```python
from build123d import *

# Parameters (mm, degrees)
F1_DEPTH = 1.5


with BuildPart() as f1:
    # F0 (on Front) → F1 (new body)
    with BuildSketch(Plane.XZ):
        with BuildLine():
            ThreePointArc((6.841464, -4), (7.649321, -2.072079), (7.925, 0))
            ThreePointArc((7.925, 0), (7.649321, 2.072079), (6.841464, 4))
            ThreePointArc((6.841464, 4), (5.603821, 5.603821), (4, 6.841464))
            ThreePointArc((4, 6.841464), (0, 7.925), (-4, 6.841464))
            ThreePointArc((-4, 6.841464), (-5.603821, 5.603821), (-6.841464, 4))
            ThreePointArc((-6.841464, 4), (-7.925, 0), (-6.841464, -4))
            ThreePointArc((-6.841464, -4), (-5.603821, -5.603821), (-4, -6.841464))
            ThreePointArc((-4, -6.841464), (0, -7.925), (4, -6.841464))
            ThreePointArc((4, -6.841464), (5.603821, -5.603821), (6.841464, -4))
        make_face()
        with BuildLine():
            ThreePointArc((-6.841464, -4), (-7.925, 0), (-6.841464, 4))
            Line((-6.841464, 4), (-9.0286, 4))
            ThreePointArc((-9.0286, 4), (-9.875, 0), (-9.0286, -4))
            Line((-9.0286, -4), (-6.841464, -4))
        make_face()
        with BuildLine():
            ThreePointArc((-4, 6.841464), (0, 7.925), (4, 6.841464))
            Line((4, 6.841464), (4, 8.629347))
            ThreePointArc((4, 8.629347), (3.895968, 8.96701), (3.619946, 9.187579))
            ThreePointArc((3.619946, 9.187579), (-0.205983, 9.872851), (-4, 9.0286))
            Line((-4, 9.0286), (-4, 6.841464))
        make_face()
        with BuildLine():
            Line((4, -9.0286), (4, -6.841464))
            ThreePointArc((4, -6.841464), (0, -7.925), (-4, -6.841464))
            Line((-4, -6.841464), (-4, -9.0286))
            ThreePointArc((-4, -9.0286), (0, -9.875), (4, -9.0286))
        make_face()
        with BuildLine():
            ThreePointArc((6.841464, 4), (7.649321, 2.072079), (7.925, 0))
            ThreePointArc((7.925, 0), (7.649321, -2.072079), (6.841464, -4))
            Line((6.841464, -4), (9.0286, -4))
            ThreePointArc((9.0286, -4), (9.872851, -0.205983), (9.187579, 3.619946))
            ThreePointArc((9.187579, 3.619946), (8.96701, 3.895968), (8.629347, 4))
            Line((8.629347, 4), (6.841464, 4))
        make_face()
    extrude(amount=F1_DEPTH)


solid = f1.part
```
The listing builds one solid part. Answer for the finished solid, in the listing's coordinates (mm). A direction names the side the tool comes from. Give positions to 0.01 mm unless a question says otherwise; leave off trailing zeros. Loops run counter-clockwise (first coordinate to the right, second up) from the corner with the lowest first, then second, coordinate; pieces in that order, holes last. Notation, with made-up numbers: M -6,49 L 20,49 A22 cw 20,73 Z; hole C -3,39.5 d6. An arc over 180 degrees is marked long. One line per item, written item: value.
Q1. A cutting plane is placed at A-A on y = -0.6. Determine the outline of the cut face in (x, z) (3 decimals).
Working result:
outline: M -9.029,-4 L -6.841,-4 A7.925 ccw -4,-6.841 L -4,-9.029 A9.875 ccw 4,-9.029 L 4,-6.841 A7.925 ccw 6.841,-4 L 9.029,-4 A9.875 ccw 9.188,3.62 A0.6 ccw 8.629,4 L 6.841,4 A7.925 ccw 4,6.841 L 4,8.629 A0.6 ccw 3.62,9.188 A9.875 ccw -4,9.029 L -4,6.841 A7.925 ccw -6.841,4 L -9.029,4 A9.875 ccw Z
Q2. Find the intervals of material crossed by line 1 (X direction, y = -1.3, z = -7.5); line 2 (X direction, y = -1.15, z = -5.25), in increasing order. Write a range as from..to.
Working result:
line 1: x = -4..4
line 2: x = -5.94..5.94
Q3. A cutting plane is placed at B-B on z = -3.25. Determine the outline of the cut face in (x, y).
Working result:
outline: M -9.32,-1.5 L 9.32,-1.5 L 9.32,0 L -9.32,0 Z
Q4. For faces 1 (the face through (-4, -1, 8)), 2 (the face through (8, -1, -4)), 3 (the face through (-8, -1, -4)), 4 (the face through (4, -1, 8)), determine the directions among +Z, -Z, +X, -X, +Y, -Y from which every point of the face is accessible in a straight line to the end or side of a thin tool.
Working result:
face 1: +Z, -X, +Y, -Y
face 2: -Z, +X, +Y, -Y
face 3: -Z, -X, +Y, -Y
face 4: +Z, +X, +Y, -Y
Q5. A cutting plane is placed at C-C on x = 8.25. Determine the outline of the cut face in (y, z), then the cut area to 3 significant figures.
Working result:
outline: M -1.5,-4 L 0,-4 L 0,4 L -1.5,4 Z
area: 12.0 mm^2
Q6. Flat-ended cylindrical pins translate along their axes: P1, Ø0.8, axis at x = -8, y = -1, coming from the +Z side; P2, Ø0.8, axis at y = -0.5, z = -7.5, coming from the +X side. Find the tip coordinate at first contact, or state that the pin passes through.
Working result:
P1: stops at z = 4
P2: stops at x = 4
